Here's how the part is built. I have some questions about the finished solid (model axes, mm). Give positions to 0.01 mm unless a question says otherwise; leave off trailing zeros. Loops run counter-clockwise (first coordinate to the right, second up) from the corner with the lowest first, then second, coordinate; pieces in that order, holes last. Notation, with made-up numbers: (64.5, 38) -> (94.5, 38) arc R5 cw to (94.5, 44) -> close; hole circle Ø5 at (18, -35). An arc over 180 degrees is marked (long way). Answer in a Markdown table with one row per item. Add a question column.
Item 1: If we section it at A-A (y = 0.45): Write out the boundary of the cut face in (x, z), then the cut area to 3 significant figures.
Item 2: If I drill on line 1 (X direction, y = 0.5, z = -2.75); line 2 (X direction, y = 0.1, z = 0) (3 decimals); line 3 (X direction, y = 0.1, z = -7) (3 decimals), over which ranges is the centre line in solid material (lowest first)?
Item 3: For P1, Ø5, axis at x = -5.5, z = 2, coming from the +Y side, with a flat end and sliding along its axis, tell me the tip position at first contact or that it passes through.
Autodesk Inventor part; units mm, degrees
ref_plane "YZ Plane" through (0, 0, 0) normal (1, 0, 0) x (0, 1, 0)
ref_plane "XZ Plane" through (0, 0, 0) normal (0, 1, 0) x (-1, 0, 0)
ref_plane "XY Plane" through (0, 0, 0) normal (0, 0, 1) x (1, 0, 0)
sketch "Boceto1" plane through (0, 0, 0) normal (0, 1, 0) x (-1, 0, 0)
  line L0 (4.925, -3.9) -> (4.925, -4.2)
  line L1 (4.925, -4.2) -> (2.025, -4.2)
  line L2 (2.025, -4.2) -> (2.025, -3.9)
  line L3 (2.025, -3.9) -> (4.925, -3.9)
  line L4 (-4.925, -3.3) -> (-2.025, -3.3)
  line L5 (-2.025, -3.3) -> (-2.025, -3.6)
  line L6 (-2.025, -3.6) -> (-4.925, -3.6)
  line L7 (-4.925, -3.6) -> (-4.925, -3.3)
  line L8 (3, 2.4695) -> (3, 2.7695)
  line L9 (3, 2.7695) -> (5.7, 2.7695)
  line L10 (5.7, 2.7695) -> (5.7, 2.4695)
  line L11 (5.7, 2.4695) -> (3, 2.4695)
  line L12 (3, 3.0695) -> (3, 3.3695)
  line L13 (3, 3.3695) -> (5.4, 3.3695)
  line L14 (5.4, 3.3695) -> (5.4, 3.0695)
  line L15 (5.4, 3.0695) -> (3, 3.0695)
  line L16 (2.025, -5.4) -> (3.825, -5.4)
  line L17 (3.825, -5.4) -> (3.825, -5.7)
  line L18 (3.825, -5.7) -> (2.025, -5.7)
  line L19 (2.025, -5.7) -> (2.025, -5.4)
  line L20 (-3.825, -5.7) -> (-3.825, -5.4)
  line L21 (-3.825, -5.4) -> (-2.025, -5.4)
  line L22 (-2.025, -5.4) -> (-2.025, -5.7)
  line L23 (-2.025, -5.7) -> (-3.825, -5.7)
  line L24 (-3.825, -6.3) -> (-3.825, -6)
  line L25 (-3.825, -6) -> (-2.025, -6)
  line L26 (-2.025, -6) -> (-2.025, -6.3)
  line L27 (-2.025, -6.3) -> (-3.825, -6.3)
  line L28 (2.025, -6.3) -> (2.025, -6)
  line L29 (2.025, -6) -> (3.825, -6)
  line L30 (3.825, -6) -> (3.825, -6.3)
  line L31 (3.825, -6.3) -> (2.025, -6.3)
  line L32 (-3, 3.3695) -> (-3, 3.0695)
  line L33 (-3, 3.0695) -> (-5.4, 3.0695)
  line L34 (-5.4, 3.0695) -> (-5.4, 3.3695)
  line L35 (-5.4, 3.3695) -> (-3, 3.3695)
  line L36 (-3, 2.7695) -> (-3, 2.4695)
  line L37 (-3, 2.4695) -> (-5.7, 2.4695)
  line L38 (-5.7, 2.4695) -> (-5.7, 2.7695)
  line L39 (-5.7, 2.7695) -> (-3, 2.7695)
  line L40 (-4.925, -4.2) -> (-4.925, -3.9)
  line L41 (-4.925, -3.9) -> (-2.025, -3.9)
  line L42 (-2.025, -3.9) -> (-2.025, -4.2)
  line L43 (-2.025, -4.2) -> (-4.925, -4.2)
  line L44 (4.925, -3.6) -> (2.025, -3.6)
  line L45 (2.025, -3.6) -> (2.025, -3.3)
  line L46 (2.025, -3.3) -> (4.925, -3.3)
  line L47 (4.925, -3.3) -> (4.925, -3.6)
  line L48 (0.15, -6.5) -> (-0.15, -6.5)
  line L49 (-1.2, -6.5) -> (-1.5, -6.5)
  line L50 (1.5, -6.5) -> (1.2, -6.5)
  line L51 (-6.725, -2.7) -> (-6.725, 1.7)
  line L52 (-6.725, 1.7) -> (-4.325, 1.7)
  line L53 (-4.325, 1.7) -> (-4.325, -2.7)
  line L54 (-4.325, -2.7) -> (-6.725, -2.7)
  line L55 (4.3, -2.7) -> (4.3, 1.7)
  line L56 (4.3, 1.7) -> (6.7, 1.7)
  line L57 (6.7, 1.7) -> (6.7, -2.7)
  line L58 (6.7, -2.7) -> (4.3, -2.7)
  circle A0 centre (-4.734, 4.334) radius 0.15
  circle A1 centre (4.734, 4.334) radius 0.15
  circle A2 centre (-4.734, -5.334) radius 0.15
  circle A3 centre (4.734, -5.334) radius 0.15
  circle A4 centre (-3.8, 0.894) radius 0.15
  circle A5 centre (-3.8, -1.894) radius 0.15
  circle A6 centre (3.8, 0.894) radius 0.15
  circle A7 centre (3.8, -1.894) radius 0.15
  line L59 (2.55, -1.4) -> (-2.55, -1.4)
  line L60 (1.5, -1.4) -> (1.5, -6.5)
  line L61 (1.2, -6.5) -> (1.2, -1.4)
  line L62 (0.15, -1.4) -> (0.15, -6.5)
  line L63 (-0.15, -6.5) -> (-0.15, -1.4)
  line L64 (-1.5, -6.5) -> (-1.5, -1.4)
  line L65 (-1.2, -1.4) -> (-1.2, -6.5)
  line L66 (2.55, -1.4) -> (2.55, 6.6532)
  line L67 (-2.55, -1.4) -> (-2.55, 6.6532)
  line L68 (-7.5, -0.5) -> (-7.5, -0.4)
  line L69 (7.5, -0.5) -> (7.5, -0.4)
  line L70 (-7.5, -0.5) -> (-7.5, -0.6)
  line L71 (7.4993, -0.5) -> (7.4993, -0.6)
  arc A8 (-7.5, -0.6) -> (7.4993, -0.6) centre (-0.0003, -0.6) ccw
  arc A9 (7.4993, -0.5) -> (2.55, 6.6532) centre (0, -0.4) ccw
  arc A10 (-2.55, 6.6532) -> (-7.5, -0.4) centre (0, -0.4) ccw
  line L72 (-4.734, -5.184) -> (-5.4457, -5.184)
  line L73 (-4.734, -5.184) -> (-4.734, -5.334)
  point P0 (2.352, 6.909)
  dimension "d13" = 0.1
  dimension "d14" = 0.1
  dimension "d15" = 0.1
extrude "Extrusión1" add sketch "Boceto1" along normal blind 0.3 contours L62 L59 L61 L50 L60 L66 A9 L69 L71 A8 L70 L68 A10 L67 L64 L49 L65 L63 L48
sketch "Boceto2" plane through (0, 0.3, 0) normal (0, 1, 0) x (1, 0, 0)
  line L0 (-1.2, 6.5) -> (-1.2, 1.4)
  line L1 (-1.5, 1.4) -> (-1.5, 6.5)
  line L2 (-0.15, 1.4) -> (-0.15, 6.5)
  line L3 (0.15, 6.5) -> (0.15, 1.4)
  line L4 (1.2, 1.4) -> (1.2, 6.5)
  line L5 (1.5, 6.5) -> (1.5, 1.4)
  line L6 (1.2, 6.5) -> (1.5, 6.5)
  line L7 (-0.15, 6.5) -> (0.15, 6.5)
  line L8 (-1.5, 6.5) -> (-1.2, 6.5)
  line L9 (-1.5, 6.5) -> (-1.2, 6.5)
  line L10 (-1.2, 6.5) -> (-1.2, 1.4)
  line L11 (-1.2, 1.4) -> (-1.5, 1.4)
  line L12 (-1.5, 1.4) -> (-1.5, 6.5)
  line L13 (-0.15, 6.5) -> (0.15, 6.5)
  line L14 (0.15, 6.5) -> (0.15, 1.4)
  line L15 (0.15, 1.4) -> (-0.15, 1.4)
  line L16 (-0.15, 1.4) -> (-0.15, 6.5)
  line L17 (1.2, 6.5) -> (1.5, 6.5)
  line L18 (1.5, 6.5) -> (1.5, 1.4)
  line L19 (1.5, 1.4) -> (1.2, 1.4)
  line L20 (1.2, 1.4) -> (1.2, 6.5)
  point P0 (0, 0)
extrude "Extrusión2" add sketch "Boceto2" along normal mid plane 0.6
sketch "Boceto3" plane through (-2.4, 0, -1.4) normal (0, 0, 1) x (1, 0, 0)
  line L0 (0, 0) -> (4.8, 0)
  line L1 (0, 0.3) -> (4.8, 0.3)
  line L2 (0, 0.3) -> (4.8, 0.3)
  line L3 (9.9, 0.3) -> (-5.1, 0.3)
  line L4 (4.8, 0) -> (0, 0)
  line L5 (9.9, 0) -> (-5.1, 0)
  line L6 (-0.3, 0.15) -> (-0.15, 0)
  line L7 (-0.3, 0.15) -> (-0.15, 0.3)
  line L8 (5.1, 0.15) -> (4.95, 0.3)
  line L9 (5.1, 0.15) -> (4.95, 0)
  line L10 (-0.15, 0.3) -> (4.95, 0.3)
  line L11 (4.95, 0) -> (-0.15, 0)
  point P0 (2.4, 0)
  point P1 (0.048, 0)
  point P2 (4.752, 0)
extrude "Extrusión3" cut sketch "Boceto3" along normal blind 10
sketch "Boceto4" plane through (0, 0.3, 0) normal (0, 1, 0) x (1, 0, 0)
  circle A0 centre (-0.675, 7) radius 0.15
  line L0 (4.325, -1.7) -> (4.325, 2.7)
  circle A1 centre (0.675, 7) radius 0.15
  line L1 (-6.7, -1.7) -> (-6.7, 2.7)
  line L2 (-6.7, 2.7) -> (-4.3, 2.7)
  line L3 (-4.3, 2.7) -> (-4.3, -1.7)
  line L4 (-4.3, -1.7) -> (-6.7, -1.7)
  line L5 (4.325, 2.7) -> (6.725, 2.7)
  line L6 (6.725, 2.7) -> (6.725, -1.7)
  line L7 (-3.825, 5.8) -> (-2.025, 5.8)
  line L8 (-2.025, 5.5) -> (-3.825, 5.5)
  line L9 (2.025, 5.8) -> (3.825, 5.8)
  line L10 (3.825, 5.5) -> (2.025, 5.5)
  line L11 (4.325, 2.7) -> (6.725, 2.7)
  line L12 (2.025, 6.3) -> (3.825, 6.3)
  point P0 (0, 0)
extrude "Extrusión4" cut sketch "Boceto4" against normal blind 10 contours A0 | A1
sketch "Boceto8" plane through (0, 0.3, 0) normal (0, 1, 0) x (1, 0, 0)
  circle A0 centre (-3.8, -0.894) radius 0.15
  line L0 (0, 0) -> (0, -2.4412)
  circle A1 centre (3.8, -0.894) radius 0.15
  circle A2 centre (3.6, 4.906) radius 0.15
  circle A3 centre (-3.6, 4.906) radius 0.15
  dimension "d33" = 0.3
  dimension "d34" = 0.3
extrude "Extrusión6" cut sketch "Boceto8" against normal blind 10 contours A2 | A3
sketch "Boceto9" plane through (0, 0, 0) normal (0, -1, 0) x (1, 0, 0)
  line L0 (-2.85, 3.6695) -> (-4.09, 3.6695)
  line L1 (-4.09, 5.5295) -> (-4.09, 3.6695)
  line L2 (-2.85, 3.6695) -> (-2.85, 5.5295)
  line L3 (-4.09, 5.5295) -> (-2.85, 5.5295)
  line L4 (-3, 3.3695) -> (-5.4, 3.3695)
  line L5 (-2.55, 6.6532) -> (-2.55, -1.4)
  point P0 (0, 0)
extrude "Extrusión7" cut sketch "Boceto9" against normal blind 10
properties part number "LBase"
Recorded:
| question | item | result |
|---|---|---|
| 1 | outline | (-1.5, -6.5) -> (-1.2, -6.5) -> (-1.2, -1.4) -> (-1.5, -1.4) -> close; (-0.15, -6.5) -> (0.15, -6.5) -> (0.15, -1.4) -> (-0.15, -1.4) -> close; (1.2, -6.5) -> (1.5, -6.5) -> (1.5, -1.4) -> (1.2, -1.4) -> close |
| 1 | area | 4.59 mm^2 |
| 2 | line 1 | x = -1.5 to -1.2, -0.15 to 0.15, 1.2 to 1.5 |
| 2 | line 2 | x = -7.49 to -6.7, -4.3 to -2.65, 2.65 to 4.325, 6.725 to 7.489 |
| 2 | line 3 | x = -3.909 to -0.825, -0.525 to 0.525, 0.825 to 3.91 |
| 3 | P1 | stops at y = 0.3 |
